Geometry check sheet. Reference: the model listing, model coordinates, mm. Give positions to 0.01 mm unless a question says otherwise; leave off trailing zeros. Write each loop counter-clockwise with the first axis right and the second up, starting at its lowest first coordinate (ties: lowest second). Pieces come first, ordered by that corner, then holes. Notation, with made-up numbers: (87, -20.75) -> (122, -20.75) arc R13 cw to (122, -5.75) -> close; hole circle Ø10 at (27, 62). An arc over 180 degrees is marked (long way). One line per item, written item: value.
from build123d import *

# Parameters (mm, degrees)
F0_R     = 15
F1_DEPTH = 21.8
F3_DEPTH = 17.5
F4_R     = 1.2
F5_DEPTH = 25.4


with BuildPart() as f1:
    # F0 (on Top) → F1 (new body)
    with BuildSketch(Plane.XY):
        Circle(F0_R)
    extrude(amount=F1_DEPTH)

    # F2 (on face) → F3 (cut)
    with BuildSketch(Plane.XY.offset(21.8)):
        with BuildLine():
            Line((0, -8.5), (0, 8.5))
            ThreePointArc((0, 8.5), (-8.5, 0), (0, -8.5))
        make_face()
        with BuildLine():
            ThreePointArc((8.5, 0), (6.010408, 6.010408), (0, 8.5))
            Line((0, 8.5), (0, -8.5))
            ThreePointArc((0, -8.5), (6.010408, -6.010408), (8.5, 0))
        make_face()
    extrude(amount=-F3_DEPTH, mode=Mode.SUBTRACT)

    # F4 (on face) → F5 (cut)
    with BuildSketch(Plane(origin=(0, 0, 0), x_dir=(1, 0, 0), z_dir=(0, 0, -1))):
        Circle(F4_R)
    extrude(amount=-F5_DEPTH, mode=Mode.SUBTRACT)


solid = f1.part
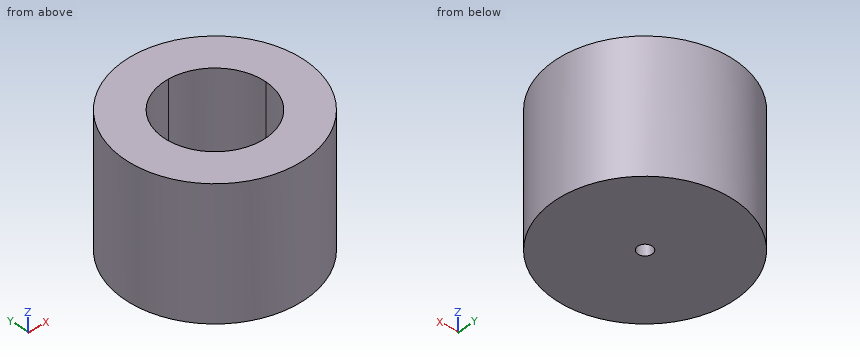
1) Sectioned sample at B-B on y = -7. Record the cut outline in (x, z), plus the area to 3 significant figures.
Verdict:
outline: (-13.27, 0) -> (13.27, 0) -> (13.27, 21.8) -> (4.82, 21.8) -> (4.82, 4.3) -> (-4.82, 4.3) -> (-4.82, 21.8) -> (-13.27, 21.8) -> close
area: 410 mm^2
2) Sectioned sample at C-C on x = -4.25. Record the cut outline in (y, z), plus the area to 3 significant figures.
Verdict:
outline: (-14.39, 0) -> (14.39, 0) -> (14.39, 21.8) -> (7.36, 21.8) -> (7.36, 4.3) -> (-7.36, 4.3) -> (-7.36, 21.8) -> (-14.39, 21.8) -> close
area: 370 mm^2
3) Depth check by flat-ended pin: pin 1 Ø1 at (x, z) = (-10.5, 14) entering from -Y; pin 2 Ø2 at (y, z) = (7, 2.5) entering from +X; pin 3 Ø4 at (x, z) = (-6.5, 6.5) entering from -Y. Enter the tip coordinate at first touch or a pass-through.
Verdict:
pin 1: y = -11.18
pin 2: x = 13.75
pin 3: y = -14.31
4) Sectioned sample at D-D on z = 16.5. Record the cut outline in (x, y).
Verdict:
outline: circle Ø30 at (0, 0); hole (0, -8.5) arc R8.5 ccw to (8.5, 0) arc R8.5 ccw to (0, 8.5) arc R8.5 ccw to start
5) Sectioned sample at A-A on z = 2.75. Record the cut outline in (x, y), plus the area to 3 significant figures.
Verdict:
outline: circle Ø30 at (0, 0); hole circle Ø2.4 at (0, 0)
area: 702 mm^2
6) Scan lines: probe 1 along Y at (x, z) = (0, 3.25); probe 2 along Y at (x, z) = (-0.25, 10.75); probe 3 along X at (y, z) = (6.5, 5). Record each from-to range of solid material in increasing order.
Verdict:
probe 1: -15 to -1.2, 1.2 to 15
probe 2: -15 to -8.5, 8.5 to 15
probe 3: -13.52 to -5.48, 5.48 to 13.52
